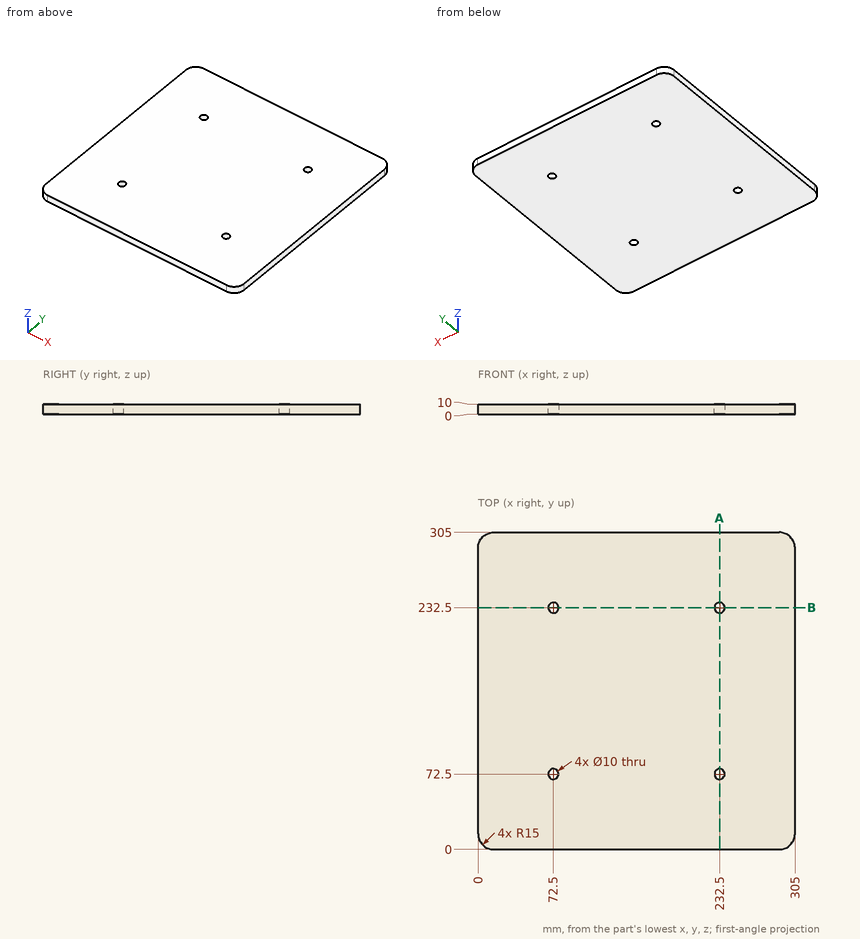
Design review of the part shown in the three views and the two pictorial views. Dimensions are in mm from the part's minimum x, y and z. Round coordinates to 2 decimals unless told otherwise and drop trailing zeros. Write each loop counter-clockwise with the first axis right and the second up, starting at its lowest first coordinate (ties: lowest second). Pieces come first, ordered by that corner, then holes. Notation, with made-up numbers: (15, 44) -> (50, 44) arc R13 ccw to (50, 54) -> close; hole circle Ø7 at (-21, -32). An arc over 180 degrees is marked (long way). Answer as a JSON object with one key per item and string values.
1. Clearance check with a flat-ended pin moving along its axis: pin 1 (9 mm diameter, centred on x = 232.5, y = 72.5, fed in from -Z). State where the tip first meets the part, or that it passes through.
Results found:
{"pin 1": "passes through"}
2. To check wall thickness, follow line 1 along Y through (x, z) = (72.5, 3.25). State the ranges of the line that lie inside material, in increasing order.
Results found:
{"line 1": "y = 0 to 67.5, 77.5 to 227.5, 237.5 to 305"}
3. We need section A-A on x = 232.5. State the section outline as (y, z) points.
Results found:
{"outline": "(0, 0) -> (67.5, 0) -> (67.5, 10) -> (0, 10) -> close; (77.5, 0) -> (227.5, 0) -> (227.5, 10) -> (77.5, 10) -> close; (237.5, 0) -> (305, 0) -> (305, 10) -> (237.5, 10) -> close"}
